```python
from build123d import *

# Parameters (mm, degrees)
F0_R     = 10.75
F1_DEPTH = 5
F2_R     = 12
F3_R     = 6


with BuildPart() as f1:
    # F0 (on Top) → F1 (new body)
    with BuildSketch(Plane.XY):
        with BuildLine():
            ThreePointArc((-10, -30), (0, -20), (10, -30))
            Line((10, -30), (51.961524, -30))
            Line((51.961524, -30), (30.980762, 6.339746))
            ThreePointArc((30.980762, 6.339746), (17.320508, 10), (20.980762, 23.660254))
            Line((20.980762, 23.660254), (0, 60))
            Line((0, 60), (-20.980762, 23.660254))
            ThreePointArc((-20.980762, 23.660254), (-17.320508, 10), (-30.980762, 6.339746))
            Line((-30.980762, 6.339746), (-51.961524, -30))
            Line((-51.961524, -30), (-10, -30))
        make_face()
        with Locations((-23.8157, -13.749997)):
            Circle(F0_R, mode=Mode.SUBTRACT)
        with Locations((23.815698, -13.750001)):
            Circle(F0_R, mode=Mode.SUBTRACT)
        Circle(F0_R, mode=Mode.SUBTRACT)
        with Locations((0, 27.5)):
            Circle(F0_R, mode=Mode.SUBTRACT)
    extrude(amount=F1_DEPTH)

    # F2
    f2_edges = [f1.edges().sort_by_distance(p)[0] for p in [
        (-51.961524, -30, 2.5),
        (51.961524, -30, 2.5),
        (0, 60, 2.5),
    ]]
    fillet(f2_edges, radius=F2_R)

    # F3
    f3_edges = [f1.edges().sort_by_distance(p)[0] for p in [
        (30.980762, 6.339746, 2.5),
        (20.980762, 23.660254, 2.5),
        (-20.980762, 23.660254, 2.5),
        (-30.980762, 6.339746, 2.5),
        (-10, -30, 2.5),
        (10, -30, 2.5),
    ]]
    fillet(f3_edges, radius=F3_R)


solid = f1.part
```
Verification items for the finished model (mm, model axes). A direction names the side the tool comes from. Give positions to 0.01 mm unless a question says otherwise; leave off trailing zeros. Order: outer loops, then holes, each group sorted by start corner. A loop starts at its lowest first (then second) coordinate and runs counter-clockwise, first axis right, second up. Notation, with made-up numbers: M 32.25,58.25 L 43.25,58.25 A23 cw 43.25,68.25 Z; hole C -13,5.5 d5. An arc over 180 degrees is marked long. Answer in a Markdown table with one row per item. Add a question column.
Item 1: Mould release check, pull along Y, two halves, no side actions. Record for faces 3 (the cylindrical face through (0, 48, 3)), 4 (the cylindrical face through (13.076, -13.277, 2.465)), 5 (the cylindrical face through (41.48, -24.15, 2.54)): released by +Y, released by -Y, zero draft, split by the parting line, or undercut.
Item 2: Section check A-A, the plane x = 0. Enter the section's corners in (y, z).
Item 3: Tool access check on faces 1 (the flat face through (-14.42, 35.02, 2.46)), 2 (the cylindrical face through (-11.52, -29.003, 2.535)). Record the directions out of +Z, -Z, +X, -X, +Y, -Y that give a thin tool (end or side, any length) a straight path to the whole face; none if there is none.
Item 4: Section check D-D, the plane z = 2.15. Enter the section's corners in (x, y), and give its area (3 significant figures).
Item 5: Gauge pin test, flat ends, axial feed: pin 1 (13 mm diameter, centred on x = 0, y = 0, fed in from +Z); pin 2 (1 mm diameter, centred on y = 33, z = 1.5, fed in from +X). Record the tip position at first contact, or that the pin passes through.
Item 6: Section check C-C, the plane y = 0. Enter the section's corners in (x, z).
Item 7: Scan lines: probe 1 along X at (y, z) = (-14.5, 1.55); probe 2 along Y at (x, z) = (2, 3.8); probe 3 along X at (y, z) = (2, 4.1). Record each from-to range of solid material in increasing order. Write a range as from..to.
Item 8: Section check B-B, the plane y = -8. Enter the section's corners in (x, z), and give its area (3 significant figures).
Filled sheet:
| question | item | result |
|---|---|---|
| 1 | face 3 | released by +Y |
| 1 | face 4 | undercut |
| 1 | face 5 | split by the parting line |
| 2 | outline | M -20,0 L -10.75,0 L -10.75,5 L -20,5 Z; M 10.75,0 L 16.75,0 L 16.75,5 L 10.75,5 Z; M 38.25,0 L 48,0 L 48,5 L 38.25,5 Z |
| 3 | face 1 | +Z, -Z, -X, +Y |
| 3 | face 2 | +Z, -Z, -Y |
| 4 | outline | M -41.57,-12 A12 ccw -31.18,-30 L -14.83,-30 A6 ccw -9.27,-26.25 A10 cw 9.27,-26.25 A6 ccw 14.83,-30 L 31.18,-30 A12 ccw 41.57,-12 L 33.4,2.15 A6 ccw 27.37,5.1 A10 cw 18.1,21.15 A6 ccw 18.56,27.85 L 10.39,42 A12 ccw -10.39,42 L -18.56,27.85 A6 ccw -18.1,21.15 A10 cw -27.37,5.1 A6 ccw -33.4,2.15 Z; hole C -23.82,-13.75 d21.5; hole C 0,0 d21.5; hole C 0,27.5 d21.5; hole C 23.82,-13.75 d21.5 |
| 4 | area | 2,430 mm^2 |
| 5 | pin 1 | passes through |
| 5 | pin 2 | stops at x = 15.88 |
| 6 | outline | M -34.64,0 L -10.75,0 L -10.75,5 L -34.64,5 Z; M 10.75,0 L 34.64,0 L 34.64,5 L 10.75,5 Z |
| 7 | probe 1 | x = -42.66..-34.54, -13.09..13.09, 34.54..42.66 |
| 7 | probe 2 | y = -20.2..-10.56, 10.56..16.94, 38.06..47.83 |
| 7 | probe 3 | x = -33.49..-10.56, 10.56..33.49 |
| 8 | outline | M -39.26,0 L -32.9,0 L -32.9,5 L -39.26,5 Z; M -14.73,0 L -7.18,0 L -7.18,5 L -14.73,5 Z; M 7.18,0 L 14.73,0 L 14.73,5 L 7.18,5 Z; M 32.9,0 L 39.26,0 L 39.26,5 L 32.9,5 Z |
| 8 | area | 139 mm^2 |
